```python
from build123d import *

# Parameters (mm, degrees)
CHAMFER1_SIZE = 0.12
CHAMFER2_SIZE = 0.2


with BuildPart() as part:
    # Sketch1 → Revolve1 (revolve)
    with BuildSketch(Plane(origin=(0, 0, 0), x_dir=(0, 0, -1), z_dir=(1, 0, 0))):
        with BuildLine():
            Line((-5, 0), (-5, 3))
            Line((-5, 3), (-0.05, 3))
            ThreePointArc((-0.05, 3), (-0.014644661, 2.985355339), (0, 2.95))
            Line((0, 2.95), (0, 2.193649167))
            ThreePointArc((0, 2.193649167), (-0.010471529, 2.163030546), (-0.0375, 2.145236875))
            ThreePointArc((-0.0375, 2.145236875), (-0.148804454, 1.981099356), (0, 1.85))
            Line((0, 1.85), (0.3, 1.85))
            Line((0.3, 1.85), (0.3, 2))
            Line((0.3, 2), (6, 2))
            Line((6, 2), (6, 0))
            Line((6, 0), (-5, 0))
        make_face()
    revolve(axis=Axis((0, 0, 12.7), (0, 0, -1)))

    # Chamfer1
    chamfer1_edges = [part.edges().sort_by_distance(p)[0] for p in [
        (0, -3, 5),
    ]]
    chamfer(chamfer1_edges, length=CHAMFER1_SIZE)

    # Chamfer2
    chamfer2_edges = [part.edges().sort_by_distance(p)[0] for p in [
        (0, -2, -6),
    ]]
    chamfer(chamfer2_edges, length=CHAMFER2_SIZE)


solid = part.part
```
Work out the finished part from the listing and answer in its coordinate system (mm). Round coordinates to 2 decimals unless told otherwise and drop trailing zeros. Write each loop counter-clockwise with the first axis right and the second up, starting at its lowest first coordinate (ties: lowest second). Pieces come first, ordered by that corner, then holes. Notation, with made-up numbers: (76.25, -26) - (96.25, -26) arc R36 ccw to (96.25, 9) - close; hole circle Ø2 at (-30.5, 50). An arc over 180 degrees is marked (long way). Return JSON: item names as keys, results as strings. Group by question number.
Q1. The part is cut by section C-C on z = 1.5. Write down the section's boundary in (x, y).
Q2. The mould has two halves that part along Z. Classify faces 1 (the cylindrical face through (-2, 0, -3)), 2 (the flat face through (0, 0, 5)), 3 (the cylindrical face through (-0.71, 1.71, -0.15)), 4 (the flat face through (0, 0, -6)): released by +Z, released by -Z, zero draft, split by the parting line, or undercut.
Q3. Find the intervals of material crossed by L1, parallel to Z at x = 2.75, y = 0; L2, parallel to Y at x = -1.5, z = -3; L3, parallel to X at y = -1, z = 2.5, in increasing order.
Q4. The part is cut by section A-A on y = 0. Write down the section's boundary in (x, z).
Q5. The part is cut by section D-D on z = -0.5. Write down the section's boundary in (x, y).
Q6. This flat-tipped pin is pushed along its axis until it touches: pin 1 Ø1.5 at (y, z) = (0, -2.5) entering from -X. Where does it stop, or does it pass through?
Solved:
{
 "1": {"outline": "circle Ø6 at (0, 0)"},
 "2": {"face 1": "zero draft", "face 2": "released by +Z", "face 3": "undercut", "face 4": "released by -Z"},
 "3": {"L1": "0 to 5", "L2": "-1.32 to 1.32", "L3": "-2.83 to 2.83"},
 "4": {"outline": "(-3, 0.05) arc R0.05 ccw to (-2.95, 0) - (-2.19, 0) arc R0.05 ccw to (-2.15, 0.04) arc R0.15 cw to (-1.85, 0) - (-1.85, -0.3) - (-2, -0.3) - (-2, -5.8) - (-1.8, -6) - (1.8, -6) - (2, -5.8) - (2, -0.3) - (1.85, -0.3) - (1.85, 0) arc R0.15 cw to (2.15, 0.04) arc R0.05 ccw to (2.19, 0) - (2.95, 0) arc R0.05 ccw to (3, 0.05) - (3, 4.88) - (2.88, 5) - (-2.88, 5) - (-3, 4.88) - close"},
 "5": {"outline": "circle Ø4 at (0, 0)"},
 "6": {"pin 1": "x = -2"}
}
